Autodesk Inventor part; units mm, degrees
ref_plane "YZ Plane" through (0, 0, 0) normal (1, 0, 0) x (0, 1, 0)
ref_plane "XZ Plane" through (0, 0, 0) normal (0, 1, 0) x (-1, 0, 0)
ref_plane "XY Plane" through (0, 0, 0) normal (0, 0, 1) x (1, 0, 0)
sketch "Sketch1" plane through (0, 0, 0) normal (1, 0, 0) x (0, 1, 0)
  line L0 (-25, 35) -> (25, 35)
  line L1 (25, 35) -> (25, -35)
  line L2 (25, -35) -> (-25, -35)
  line L3 (-25, -35) -> (-25, 35)
  line L4 (-25, 35) -> (25, -35) construction
  line L5 (25, 35) -> (-25, -35) construction
  point P0 (0, 0)
  dimension "d0" = 50
  dimension "d1" = 70
extrude "Extrusion1" add sketch "Sketch1" along normal blind 16
sketch "Sketch2" plane through (16, 0, 0) normal (1, 0, 0) x (0, 0, -1)
  circle A0 centre (0, 0) radius 15.25
  dimension "d4" = 30.5
extrude "Extrusion2" cut sketch "Sketch2" against normal through all
sketch "Sketch3" plane through (16, 0, 0) normal (1, 0, 0) x (0, 0, -1)
  circle A0 centre (0, 0) radius 15.25
  circle A1 centre (0, 0) radius 12.75
  dimension "d7" = 25.5
extrude "Extrusion3" add sketch "Sketch3" against normal blind 8
sketch "Sketch4" plane through (0, -25, 35) normal (0, 0, 1) x (1, 0, 0)
  line L0 (0, 50) -> (0, 0)
  line L1 (0, 0) -> (16, 0)
  line L2 (16, 50) -> (16, 0)
  line L3 (0, 50) -> (16, 50)
  line L4 (16, 37.75) -> (16, 12.25)
  line L5 (8, 12.25) -> (8, 37.75)
  line L6 (16, 37.75) -> (16, 12.25)
  line L7 (16, 50) -> (-64, 50)
  line L8 (-64, 50) -> (-64, -52.5)
  line L9 (-64, -52.5) -> (16, -52.5)
  line L10 (16, -52.5) -> (16, 50)
  line L11 (0, 50) -> (-64, -52.5)
  line L12 (16, 0) -> (-14, -52.5)
  point P0 (0, 25)
  point P1 (8, 25)
  dimension "d10" = 77.5
  dimension "d11" = 80
  dimension "d12" = 50
extrude "Extrusion4" add sketch "Sketch4" against normal blind 10 contours L0 L1 L12 L9 L11
mirror "Mirror1" about plane through (0, 0, 0) normal (0, 0, 1) of "Extrusion4"
sketch "Sketch5" plane through (-64, -77.5, 35) normal (0, -1, 0) x (1, 0, 0)
  line L0 (0, 0) -> (50, 0)
  line L1 (0, 0) -> (0, -10)
  line L2 (50, -10) -> (0, -10)
  line L3 (50, 0) -> (50, -10)
  line L4 (0, -70) -> (50, -70)
  line L5 (50, -70) -> (50, -60)
  line L6 (50, -60) -> (0, -60)
  line L7 (0, -70) -> (0, -60)
  line L8 (0, 0) -> (50, 0)
  line L9 (50, 0) -> (50, -70)
  line L10 (50, -70) -> (0, -70)
  line L11 (0, -70) -> (0, 0)
  point P0 (64, -35)
extrude "Extrusion5" add sketch "Sketch5" against normal blind 12
sketch "Sketch6" plane through (-64, -65.5, 35) normal (0, 1, 0) x (1, 0, 0)
  line L0 (50, 10) -> (7.4927, 10)
  line L1 (50, 10) -> (50, 60)
  line L2 (7.4927, 60) -> (50, 60)
  line L3 (7.4927, 70) -> (7.4927, 60)
  line L4 (7.4927, 70) -> (0, 70)
  line L5 (0, 70) -> (0, 0)
  line L6 (0, 0) -> (7.4927, 0)
  line L7 (7.4927, 10) -> (7.4927, 0)
  line L8 (64, 70) -> (7.4927, 70)
  line L9 (64, 70) -> (80, 70)
  line L10 (50, 70) -> (80, 70)
  line L11 (0, 70) -> (50, 70)
  line L12 (7.4927, 70) -> (0, 70)
  line L13 (50, 0) -> (80, 0)
  line L14 (64, 0) -> (80, 0)
  line L15 (64, 0) -> (7.4927, 0)
  line L16 (0, 0) -> (7.4927, 0)
  line L17 (0, 0) -> (50, 0)
  line L18 (50, 0) -> (0, 70) construction
  line L19 (50, 70) -> (0, 0) construction
  line L20 (10, 20) -> (40, 20) construction
  line L21 (40, 20) -> (40, 50) construction
  line L22 (40, 50) -> (10, 50) construction
  line L23 (10, 50) -> (10, 20) construction
  line L24 (10, 20) -> (40, 50) construction
  line L25 (40, 20) -> (10, 50) construction
  point P0 (64, 35)
  point P1 (25, 35)
  dimension "d17" = 30
  dimension "d18" = 30
hole "Hole1" at (-24, -65.5, -15) at (-54, -65.5, -15) at (-54, -65.5, 15) at (-24, -65.5, 15) direction (0, -1, 0) diameter 6.6 end through all
properties part number "Part15_3DPrint"
Here's how the part is built. I have some questions about the finished solid (model axes, mm). A direction names the side the tool comes from. Give positions to 0.01 mm unless a question says otherwise; leave off trailing zeros. Loops run counter-clockwise (first coordinate to the right, second up) from the corner with the lowest first, then second, coordinate; pieces in that order, holes last. Notation, with made-up numbers: M -39,-16.75 L -1,-16.75 A14 cw -1,-5.75 Z; hole C 54.25,11.25 d5. An arc over 180 degrees is marked long. Use one line per item in the form item = value. Start each with the question number.
Q1. If we section it at C-C (x = -24): Write out the boundary of the cut face in (y, z).
Q2. If we section it at D-D (z = 22): Write out the boundary of the cut face in (x, y), then the cut area to 3 significant figures.
Q3. If we section it at B-B (y = -45.5): Write out the boundary of the cut face in (x, z), then the cut area to 3 significant figures.
Q4. I need wall thicknesses on line 1 along Z through (x, y) = (-54, -71.5); line 2 along X through (y, z) = (-71, 15); line 3 along Z through (x, y) = (-5, -33). Which ranges of each line are inside material? Lowest first, please.
Q5. If we section it at A-A (z = 0): Write out the boundary of the cut face in (x, y), then the cut area to 3 significant figures.
Q6. Will these pins go through, and if not, where does the flat tip stop? pin 1 Ø17.5 at (x, z) = (11.5, -4) entering from -Y; pin 2 Ø4 at (y, z) = (13, -3) entering from -X; pin 3 Ø8 at (x, z) = (-26, -18.5) entering from +Y.
Q7. Thinking about a two-plate mould opening in Y: for faces 3 (the flat face through (-28.649, -20.883, -30.07)), 4 (the flat face through (0, -11, 11)), 5 (the cylindrical face through (12.056, -12.447, 2.764)), which applies, +Y half, -Y half, draft (parallel to the pull), parting line (faces both ways), or undercut?
Q8. Which directions (+Z, -Z, +X, -X, +Y, -Y) give clear straight access to the entire face, cutting with the end or side of a thin tool? Please do faces 1 (the flat face through (-27.86, -19.62, 30.07)), 2 (the flat face through (8, -11, -7)).
Taken from the geometry:
q1.outline = M -77.5,-35 L -13.44,-35 L -13.44,-25 L -65.5,-25 L -65.5,-18.3 L -77.5,-18.3 Z; M -77.5,-11.7 L -65.5,-11.7 L -65.5,11.7 L -77.5,11.7 Z; M -77.5,18.3 L -65.5,18.3 L -65.5,25 L -13.44,25 L -13.44,35 L -77.5,35 Z
q2.outline = M -64,-77.5 L -14,-77.5 L -14,-65.5 L -64,-65.5 Z; M 0,-25 L 16,-25 L 16,25 L 0,25 Z
q2.area = 1,400 mm^2
q3.outline = M -44.02,-35 L 4.29,-35 L 4.29,-25 L -44.02,-25 Z; M -44.02,25 L 4.29,25 L 4.29,35 L -44.02,35 Z
q3.area = 966 mm^2
q4.line_1 = -35 to -18.3, -11.7 to 11.7, 18.3 to 35
q4.line_2 = -64 to -57.3, -50.7 to -27.3, -20.7 to -14
q4.line_3 = -35 to -25, 25 to 35
q5.outline = M -64,-77.5 L -14,-77.5 L -14,-65.5 L -64,-65.5 Z; M 0,-25 L 16,-25 L 16,-12.75 L 8,-12.75 L 8,-15.25 L 0,-15.25 Z; M 0,15.25 L 8,15.25 L 8,12.75 L 16,12.75 L 16,25 L 0,25 Z
q5.area = 952 mm^2
q6.pin_1 = -25
q6.pin_2 = 0
q6.pin_3 = -65.5
q7.face_3 = +Y half
q7.face_4 = draft
q7.face_5 = undercut
q8.face_1 = +Z, -Z, -X, +Y
q8.face_2 = -X
